from build123d import *

# Parameters (mm, degrees)
F1_DEPTH     = 18
F3_R         = 2.1
F4_DEPTH     = 25
F5_R         = 14.99999
F6_T1_DEPTH  = 90.00002
F6_T3_DEPTH  = 46.00002
F6_T5_DEPTH  = 12.50001
F6_T7_DEPTH  = 25.50001
F6_T10_ANGLE = 90
F6_T12_ANGLE = 90
F6_T14_ANGLE = 90
F6_T16_ANGLE = 90
F6_T18_ANGLE = 90
F6_T20_ANGLE = 90
F6_T22_ANGLE = 90
F6_T24_ANGLE = 90


# Not quite as in the source:
# - a fillet or chamfer that OpenCascade refuses, or shapes differently, is made with other operations: its cross-section is extruded or revolved along the edge and cut away or added
# - a fillet or chamfer is up to 0.001 mm smaller than in the source, because OpenCascade refuses the exact size


with BuildPart() as f1:
    # F0 (on Right) → F1 (new body)
    with BuildSketch(Plane.YZ):
        Polygon((-60, 28), (-60, 0), (0, 0), (60, 0), (60, 28), (38, 28), (38, 13), (-38, 13), (-38, 28), align=None)
    extrude(amount=F1_DEPTH)

    # F3 (on offset) → F4 (cut)
    with BuildSketch(Plane.XY.offset(28)):
        with Locations((9, 48.35)):
            Circle(F3_R)
        with Locations((9, -48.35)):
            Circle(F3_R)
    extrude(amount=-F4_DEPTH, mode=Mode.SUBTRACT)

    # F5 (radius 15 in the source; OpenCascade refuses exactly that, so slightly less here)
    f5_edges = [f1.edges().sort_by_distance(p)[0] for p in [
        (9, 60, 0),
        (9, -60, 0),
        (9, -38, 13),
        (9, 38, 13),
    ]]
    fillet(f5_edges, radius=F5_R)

    # F6: fillet of radius 5 on 4 edges, made by hand

    # F6_s2 → F6_t1 (cut)
    with BuildSketch(Plane.XZ.offset(-45.00001)):
        with BuildLine():
            ThreePointArc((0, 5), (1.4644660941, 1.4644660941), (5, 0))
            Line((5, 0), (0, 0))
            Line((0, 0), (0, 5))
        make_face()
        with BuildLine():
            ThreePointArc((18, 5), (16.5355339059, 1.4644660941), (13, 0))
            Line((13, 0), (18, 0))
            Line((18, 0), (18, 5))
        make_face()
    extrude(amount=F6_T1_DEPTH, mode=Mode.SUBTRACT)

    # F6_s4 → F6_t3 (cut)
    with BuildSketch(Plane.XZ.offset(-23.00001)):
        with BuildLine():
            ThreePointArc((0, 8), (1.4644660941, 11.5355339059), (5, 13))
            Line((5, 13), (0, 13))
            Line((0, 13), (0, 8))
        make_face()
        with BuildLine():
            ThreePointArc((18, 8), (16.5355339059, 11.5355339059), (13, 13))
            Line((13, 13), (18, 13))
            Line((18, 13), (18, 8))
        make_face()
    extrude(amount=F6_T3_DEPTH, mode=Mode.SUBTRACT)

    # F6_s6 → F6_t5 (cut)
    with BuildSketch(Plane.XY.offset(27.99999)):
        with BuildLine():
            ThreePointArc((18, -43), (16.5355339059, -39.4644660941), (13, -38))
            Line((13, -38), (18, -38))
            Line((18, -38), (18, -43))
        make_face()
        with BuildLine():
            ThreePointArc((18, 43), (16.5355339059, 39.4644660941), (13, 38))
            Line((13, 38), (18, 38))
            Line((18, 38), (18, 43))
        make_face()
        with BuildLine():
            ThreePointArc((0, -43), (1.4644660941, -39.4644660941), (5, -38))
            Line((5, -38), (0, -38))
            Line((0, -38), (0, -43))
        make_face()
        with BuildLine():
            ThreePointArc((0, 43), (1.4644660941, 39.4644660941), (5, 38))
            Line((5, 38), (0, 38))
            Line((0, 38), (0, 43))
        make_face()
    extrude(amount=F6_T5_DEPTH, mode=Mode.SUBTRACT)

    # F6_s8 → F6_t7 (cut)
    with BuildSketch(Plane.XY.offset(14.99999)):
        with BuildLine():
            ThreePointArc((13, -60), (16.5355339059, -58.5355339059), (18, -55))
            Line((18, -55), (18, -60))
            Line((18, -60), (13, -60))
        make_face()
        with BuildLine():
            ThreePointArc((18, 55), (16.5355339059, 58.5355339059), (13, 60))
            Line((13, 60), (18, 60))
            Line((18, 60), (18, 55))
        make_face()
        with BuildLine():
            ThreePointArc((0, 55), (1.4644660941, 58.5355339059), (5, 60))
            Line((5, 60), (0, 60))
            Line((0, 60), (0, 55))
        make_face()
        with BuildLine():
            ThreePointArc((5, -60), (1.4644660941, -58.5355339059), (0, -55))
            Line((0, -55), (0, -60))
            Line((0, -60), (5, -60))
        make_face()
    extrude(amount=F6_T7_DEPTH, mode=Mode.SUBTRACT)

    # F6_s9 → F6_t10 (revolve, cut)
    with BuildSketch(Plane.XY.offset(27.99999)):
        with BuildLine():
            ThreePointArc((18, 43), (16.5355339059, 39.4644660941), (13, 38))
            Line((13, 38), (18, 38))
            Line((18, 38), (18, 43))
        make_face()
    revolve(axis=Axis((18, 23.00001, 27.99999), (-1, 0, 0)), revolution_arc=F6_T10_ANGLE, mode=Mode.SUBTRACT)

    # F6_s11 → F6_t12 (revolve, cut)
    with BuildSketch(Plane.XY.offset(27.99999)):
        with BuildLine():
            ThreePointArc((18, -43), (16.5355339059, -39.4644660941), (13, -38))
            Line((13, -38), (18, -38))
            Line((18, -38), (18, -43))
        make_face()
    revolve(axis=Axis((18, -23.00001, 27.99999), (1, 0, 0)), revolution_arc=F6_T12_ANGLE, mode=Mode.SUBTRACT)

    # F6_s13 → F6_t14 (revolve, cut)
    with BuildSketch(Plane.XY.offset(27.99999)):
        with BuildLine():
            ThreePointArc((0, 43), (1.4644660941, 39.4644660941), (5, 38))
            Line((5, 38), (0, 38))
            Line((0, 38), (0, 43))
        make_face()
    revolve(axis=Axis((0, 23.00001, 27.99999), (-1, 0, 0)), revolution_arc=F6_T14_ANGLE, mode=Mode.SUBTRACT)

    # F6_s15 → F6_t16 (revolve, cut)
    with BuildSketch(Plane.XY.offset(27.99999)):
        with BuildLine():
            ThreePointArc((0, -43), (1.4644660941, -39.4644660941), (5, -38))
            Line((5, -38), (0, -38))
            Line((0, -38), (0, -43))
        make_face()
    revolve(axis=Axis((0, -23.00001, 27.99999), (1, 0, 0)), revolution_arc=F6_T16_ANGLE, mode=Mode.SUBTRACT)

    # F6_s17 → F6_t18 (revolve, cut)
    with BuildSketch(Plane.XZ.offset(-45.00001)):
        with BuildLine():
            ThreePointArc((18, 5), (16.5355339059, 1.4644660941), (13, 0))
            Line((13, 0), (18, 0))
            Line((18, 0), (18, 5))
        make_face()
    revolve(axis=Axis((18, 45.00001, 14.99999), (1, 0, 0)), revolution_arc=F6_T18_ANGLE, mode=Mode.SUBTRACT)

    # F6_s19 → F6_t20 (revolve, cut)
    with BuildSketch(Plane.XY.offset(14.99999)):
        with BuildLine():
            ThreePointArc((13, -60), (16.5355339059, -58.5355339059), (18, -55))
            Line((18, -55), (18, -60))
            Line((18, -60), (13, -60))
        make_face()
    revolve(axis=Axis((18, -45.00001, 14.99999), (1, 0, 0)), revolution_arc=F6_T20_ANGLE, mode=Mode.SUBTRACT)

    # F6_s21 → F6_t22 (revolve, cut)
    with BuildSketch(Plane.XY.offset(14.99999)):
        with BuildLine():
            ThreePointArc((0, -55), (1.4644660941, -58.5355339059), (5, -60))
            Line((5, -60), (0, -60))
            Line((0, -60), (0, -55))
        make_face()
    revolve(axis=Axis((0, -45.00001, 14.99999), (1, 0, 0)), revolution_arc=F6_T22_ANGLE, mode=Mode.SUBTRACT)

    # F6_s23 → F6_t24 (revolve, cut)
    with BuildSketch(Plane.XZ.offset(-45.00001)):
        with BuildLine():
            ThreePointArc((0, 5), (1.4644660941, 1.4644660941), (5, 0))
            Line((5, 0), (0, 0))
            Line((0, 0), (0, 5))
        make_face()
    revolve(axis=Axis((0, 45.00001, 14.99999), (1, 0, 0)), revolution_arc=F6_T24_ANGLE, mode=Mode.SUBTRACT)


solid = f1.part
Geometry check sheet. Reference: the model listing, model coordinates, mm. A direction names the side the tool comes from. Round coordinates to 2 decimals unless told otherwise and drop trailing zeros. Write each loop counter-clockwise with the first axis right and the second up, starting at its lowest first coordinate (ties: lowest second). Pieces come first, ordered by that corner, then holes.
Item 1: Material ranges on line 1 along Y through (x, z) = (9, 9); line 2 along Y through (x, z) = (9, 12.75); line 3 along X through (y, z) = (48.5, 17.75), recorded low to high.
Determined:
line 1: y = -58.75 to -50.45, -46.25 to 46.25, 50.45 to 58.75
line 2: y = -59.83 to -50.45, -46.25 to 46.25, 50.45 to 59.83
line 3: x = 0 to 6.91, 11.09 to 18
Item 2: Mould release check, pull along Y, two halves, no side actions. Record for faces 4 (the face through (9.06, 55.49, 4.28)), 5 (the face through (0, -1, 6)), 6 (the face through (9.06, -55.72, 4.51)), 7 (the face through (9.06, -33.72, 17.51)): +Y half, -Y half, draft (parallel to the pull), parting line (faces both ways), or undercut.
Determined:
face 4: +Y half
face 5: draft
face 6: -Y half
face 7: undercut
Item 3: Go/stop test with flat-tipped pins: pin 1 Ø6 at (x, y) = (15.5, -32) entering from +Z; pin 2 Ø3 at (x, y) = (15, 36) entering from -Z; pin 3 Ø9 at (x, y) = (9.5, -1.5) entering from +Z. Record where each tip stops, or that it passes through.
Determined:
pin 1: stops at z = 18.41
pin 2: stops at z = 0.03
pin 3: stops at z = 13
Item 4: Access from +Z, -Z, +X, -X, +Y, -Y to the whole of each face (thin tool, end or side, straight path). Record for faces 1 (the face through (6.9, 49.2, 28)), 2 (the face through (8.54, 46.3, 15.68)), 3 (the face through (9.06, 33.72, 17.51)).
Determined:
face 1: +Z, +X, -X, +Y, -Y
face 2: +Z
face 3: +Z, +X, -X
Item 5: Section check C-C (y = -14). Record the boundary of the cut face in (x, z).
Determined:
outline: (0, 5) arc R5 ccw to (5, 0) - (13, 0) arc R5 ccw to (18, 5) - (18, 8) arc R5 ccw to (13, 13) - (5, 13) arc R5 ccw to (0, 8) - close
Item 6: Section check A-A (z = 16). Give the number of separate pieces and of enclosed holes in the cut face, plus the area to 3 significant figures.
Determined:
separate pieces: 2
enclosed holes: 2
area: 926 mm2
